Verification items for the finished model (mm, model axes). Face numbers are marked on the shaded views. Round coordinates to 2 decimals unless told otherwise and drop trailing zeros. Order: outer loops, then holes, each group sorted by start corner. A loop starts at its lowest first (then second) coordinate and runs counter-clockwise, first axis right, second up. Notation, with made-up numbers: M 79,43.25 L 119,43.25 A28 ccw 119,68.25 Z; hole C -9.75,8 d3. An arc over 180 degrees is marked long. Use one line per item in the form item = value. Start each with the question number.
Item 1: Go/stop test with a flat-tipped pin: pin 1 Ø2 at (x, y) = (-1.5, -0.5) entering from -Z. Record where the tip stops, or that it passes through.
Item 2: Thickness scan on probe 1 along X at (y, z) = (-0.45, 0); probe 2 along Z at (x, y) = (-2, 0.25); probe 3 along Z at (x, y) = (-0.25, 0.75). Record the ranges inside material, lowest first. Write a range as [from, to].
Item 3: Release check for a two-part mould opening along Z. For the marked faces 1, 2 and 3 record: +Z half, -Z half, draft (parallel to the pull), parting line (faces both ways), or undercut.
Item 4: Cross-section at A-A on y = -2. Enter the section's corners in (x, z), then the cut area to 3 significant figures.
from build123d import *

# Parameters (mm, degrees)
SKETCH3_R           = 3
BOSS_EXTRUDE1_DEPTH = 3


with BuildPart() as part:
    # Sketch3 → Boss-Extrude1 (new, symmetric)
    with BuildSketch(Plane(origin=(0, 0, 0), x_dir=(1, 0, 0), z_dir=(0, 1, 0))):
        Polygon((5, 2.886751346), (0, 5.773502692), (-5, 2.886751346), (-5, -2.886751346), (0, -5.773502692), (5, -2.886751346), align=None)
        Circle(SKETCH3_R, mode=Mode.SUBTRACT)
    extrude(amount=BOSS_EXTRUDE1_DEPTH, both=True)

    # Sketch5 → Cut-Revolve1 (revolve, cut)
    with BuildSketch(Plane(origin=(0, 0, 0), x_dir=(0, 0, -1), z_dir=(1, 0, 0))):
        with BuildLine():
            Line((3, 3), (5.773502692, 3))
            Line((5.773502692, 3), (5.773502692, 1.143539601))
            ThreePointArc((5.773502692, 1.143539601), (4.668739224, 2.493052226), (3, 3))
        make_face()
    revolve(axis=Axis((0, 0, 0), (0, 1, 0)), mode=Mode.SUBTRACT)


solid = part.part
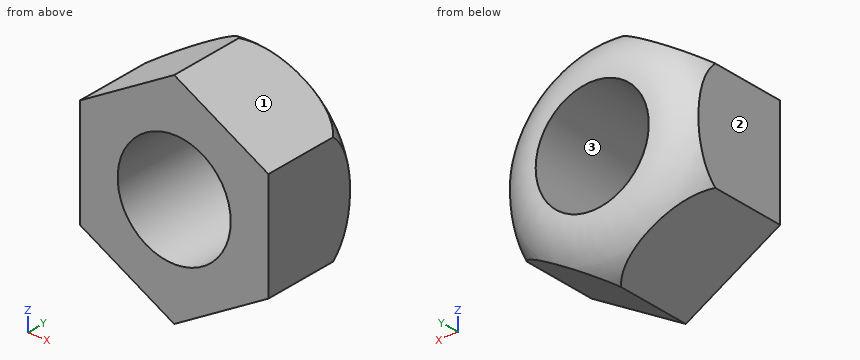
Output values:
q1.pin_1 = -5.48
q2.probe_1 = [-5, -3], [3, 5]
q2.probe_2 = [-4.62, -2.24], [2.24, 4.62]
q2.probe_3 = [-5.63, -2.99], [2.99, 5.63]
q3.face_1 = +Z half
q3.face_2 = draft
q3.face_3 = undercut
q4.outline = M -5,-2.89 L 0,-5.77 L 5,-2.89 L 5,2.89 L 0,5.77 L -5,2.89 Z; hole C 0,0 d6
q4.area = 58.3 mm2
